from build123d import *

# Parameters (mm, degrees)
CROQUIS1_R              = 42.5
SALIENTE_EXTRUIR1_DEPTH = 142
CROQUIS2_R              = 42.5
SALIENTE_EXTRUIR2_DEPTH = 52.5
CROQUIS3_R              = 42.5
CROQUIS3_R_2            = 36.143595246
CROQUIS3_R_3            = 2.508178933
SALIENTE_EXTRUIR3_DEPTH = 2
CORTAR_EXTRUIR1_START   = -25
CROQUIS6_R              = 42.5
CROQUIS6_R_2            = 41.546105734
CORTAR_EXTRUIR1_DEPTH   = 3
CORTAR_EXTRUIR2_START   = -40
CROQUIS7_R              = 42.5
CROQUIS7_R_2            = 41.546105734
CORTAR_EXTRUIR2_DEPTH   = 1
CORTAR_EXTRUIR3_START   = -30
CROQUIS8_R              = 7.355169738
CORTAR_EXTRUIR3_DEPTH   = 21


with BuildPart() as part:
    # Croquis1 → Saliente-Extruir1 (new body)
    with BuildSketch(Plane(origin=(0, 0, 0), x_dir=(1, 0, 0), z_dir=(0, 1, 0))):
        with Locations(Location((0, 0, 0), (0, 0, 270))):
            Circle(CROQUIS1_R)
    extrude(amount=SALIENTE_EXTRUIR1_DEPTH)

    # Croquis2 → Saliente-Extruir2 (add)
    with BuildSketch(Plane(origin=(0, 0, 0), x_dir=(0, 0, -1), z_dir=(1, 0, 0))):
        with Locations((0, 96)):
            Circle(CROQUIS2_R)
    extrude(amount=SALIENTE_EXTRUIR2_DEPTH)

    # Croquis3 → Saliente-Extruir3 (add)
    with BuildSketch(Plane(origin=(0, 142, 0), x_dir=(1, 0, 0), z_dir=(0, 1, 0))):
        with Locations(Location((0, 0, 0), (0, 0, 270))):
            Circle(CROQUIS3_R)
        with Locations(Location((0, 0, 0), (0, 0, 270))):
            Circle(CROQUIS3_R_2, mode=Mode.SUBTRACT)
        with Locations(Location((0, 39.319059372, 0), (0, 0, 270))):
            Circle(CROQUIS3_R_3, mode=Mode.SUBTRACT)
        with Locations(Location((34.051304269, 19.659529686, 0), (0, 0, 270))):
            Circle(CROQUIS3_R_3, mode=Mode.SUBTRACT)
        with Locations(Location((34.051304269, -19.659529686, 0), (0, 0, 270))):
            Circle(CROQUIS3_R_3, mode=Mode.SUBTRACT)
        with Locations(Location((0, -39.319059372, 0), (0, 0, 270))):
            Circle(CROQUIS3_R_3, mode=Mode.SUBTRACT)
        with Locations(Location((-34.051304269, -19.659529686, 0), (0, 0, 270))):
            Circle(CROQUIS3_R_3, mode=Mode.SUBTRACT)
        with Locations(Location((-34.051304269, 19.659529686, 0), (0, 0, 270))):
            Circle(CROQUIS3_R_3, mode=Mode.SUBTRACT)
    extrude(amount=SALIENTE_EXTRUIR3_DEPTH)

    # Croquis6 → Cortar-Extruir1 (cut)
    with BuildSketch(Plane.XZ.offset(CORTAR_EXTRUIR1_START)):
        with Locations(Location((0, 0, 0), (0, 0, 270))):
            Circle(CROQUIS6_R)
        with Locations(Location((0, 0, 0), (0, 0, 270))):
            Circle(CROQUIS6_R_2, mode=Mode.SUBTRACT)
    extrude(amount=-CORTAR_EXTRUIR1_DEPTH, mode=Mode.SUBTRACT)

    # Croquis7 → Cortar-Extruir2 (cut)
    with BuildSketch(Plane(origin=(0, 0, 0), x_dir=(-1, 0, 0), z_dir=(0, -1, 0)).offset(CORTAR_EXTRUIR2_START)):
        with Locations(Location((0, 0, 0), (0, 0, 90))):
            Circle(CROQUIS7_R)
        with Locations(Location((0, 0, 0), (0, 0, 90))):
            Circle(CROQUIS7_R_2, mode=Mode.SUBTRACT)
    extrude(amount=-CORTAR_EXTRUIR2_DEPTH, mode=Mode.SUBTRACT)

    # Croquis8 → Cortar-Extruir3 (cut)
    with BuildSketch(Plane.XY.offset(CORTAR_EXTRUIR3_START)):
        with Locations((0, 12.368172151)):
            Circle(CROQUIS8_R)
    extrude(amount=-CORTAR_EXTRUIR3_DEPTH, mode=Mode.SUBTRACT)


solid = part.part
For this review, take the finished solid that the model builds, in its own axes (mm). A direction names the side the tool comes from. Round coordinates to 2 decimals unless told otherwise and drop trailing zeros. Loops run counter-clockwise (first coordinate to the right, second up) from the corner with the lowest first, then second, coordinate; pieces in that order, holes last. Notation, with made-up numbers: (7.5, -25.75) - (41.5, -25.75) arc R20 ccw to (41.5, 9.25) - close; hole circle Ø8 at (22.5, -16). An arc over 180 degrees is marked (long way). One line per item, written item: value. Start each with the question number.
Item 1: For faces 5 (the cylindrical face through (33.091, 142.986, 21.976)), 6 (the flat face through (22, 144, -29)), 7 (the flat face through (-41, 28, -9)), list the 3-axis set-ups (+Z, -Z, +X, -X, +Y, -Y) from which the entire face can be reached by the end or side of a thin tool; tool diameter is ignored.
Item 2: Clearance check with flat-ended pins moving along their axes: pin 1 Ø2.5 at (x, z) = (35, -20) entering from +Y; pin 2 Ø6.5 at (x, z) = (34.05, -19.66) entering from -Y; pin 3 Ø6 at (y, z) = (99.5, 23.5) entering from -X; pin 4 Ø1 at (y, z) = (55, -19) entering from -X. State where each tip first meets the part, or that it passes through.
Item 3: Take a section at C-C (y = 96). Give the boundary of the cut face in (x, z).
Item 4: Take a section at B-B (x = -25.5). Give the boundary of the cut face in (y, z), plus the area to 3 significant figures.
Item 5: Take a section at D-D (z = -15). Give the boundary of the cut face in (x, y), plus the area to 3 significant figures.
Item 6: The part is to be moulded in two halves that separate along Y. For faces 1 (the flat face through (0, 12, -30)), 2 (the cylindrical face through (37.55, 97.87, 42.46)), 3 (the cylindrical face through (-25.861, 33.916, -33.727)), 4 (the cylindrical face through (-1.594, 5.188, -36.162)), say which applies: +Y half, -Y half, draft (parallel to the pull), parting line (faces both ways), or undercut.
Item 7: For L1, parallel to Y at x = 0, z = -39.5; L2, parallel to X at y = 38.5, z = 7.5; L3, parallel to Y at x = -25.5, z = 7.5, list the stretches that pass through material, from the lowest coordinate up.
Item 8: Take a section at A-A (z = 0). Give the boundary of the cut face in (x, y), plus the area to 3 significant figures.
Answer below:
1. face 5: +Y
1. face 6: +Z, -Z, +X, -X, +Y
1. face 7: none
2. pin 1: stops at y = 142
2. pin 2: stops at y = 0
2. pin 3: stops at x = -37.23
2. pin 4: stops at x = -38.26
3. outline: (0, -42.5) - (52.5, -42.5) - (52.5, 42.5) - (0, 42.5) arc R42.5 ccw to start
4. outline: (0, -34) - (25, -34) - (25, -32.8) - (28, -32.8) - (28, -34) - (40, -34) - (40, -32.8) - (41, -32.8) - (41, -34) - (144, -34) - (144, -25.61) - (142, -25.61) - (142, 25.61) - (144, 25.61) - (144, 34) - (41, 34) - (41, 32.8) - (40, 32.8) - (40, 34) - (28, 34) - (28, 32.8) - (25, 32.8) - (25, 34) - (0, 34) - close
4. area: 9,680 mm2
5. outline: (-39.76, 0) - (39.76, 0) - (39.76, 25) - (38.74, 25) - (38.74, 28) - (39.76, 28) - (39.76, 40) - (38.74, 40) - (38.74, 41) - (39.76, 41) - (39.76, 56.24) - (52.5, 56.24) - (52.5, 135.76) - (39.76, 135.76) - (39.76, 144) - (32.88, 144) - (32.88, 142) - (-32.88, 142) - (-32.88, 144) - (-39.76, 144) - (-39.76, 41) - (-38.74, 41) - (-38.74, 40) - (-39.76, 40) - (-39.76, 28) - (-38.74, 28) - (-38.74, 25) - (-39.76, 25) - close
5. area: 12,300 mm2
6. face 1: undercut
6. face 2: parting line
6. face 3: draft
6. face 4: undercut
7. L1: y = 0 to 5.01, 19.72 to 142
7. L2: x = -41.83 to 41.83
7. L3: y = 0 to 142
8. outline: (-42.5, 0) - (42.5, 0) - (42.5, 25) - (41.55, 25) - (41.55, 28) - (42.5, 28) - (42.5, 40) - (41.55, 40) - (41.55, 41) - (42.5, 41) - (42.5, 53.5) - (52.5, 53.5) - (52.5, 138.5) - (42.5, 138.5) - (42.5, 144) - (36.14, 144) - (36.14, 142) - (-36.14, 142) - (-36.14, 144) - (-42.5, 144) - (-42.5, 41) - (-41.55, 41) - (-41.55, 40) - (-42.5, 40) - (-42.5, 28) - (-41.55, 28) - (-41.55, 25) - (-42.5, 25) - close
8. area: 12,900 mm2
